```python
from build123d import *

# Parameters (mm, degrees)
BOSS_EXTRUDE1_DEPTH = 3.18
CUT_EXTRUDE1_DEPTH  = 3.18
SKETCH3_W           = 42
SKETCH3_H           = 20
CUT_EXTRUDE2_DEPTH  = 10
SKETCH4_R           = 2.2225
CUT_EXTRUDE3_DEPTH  = 10
SKETCH5_R           = 8.5
SKETCH5_W           = 12
SKETCH5_H           = 3.600941215
CUT_EXTRUDE4_DEPTH  = 10
SKETCH6_R           = 1.2
CUT_EXTRUDE5_DEPTH  = 10


with BuildPart() as part:
    # Sketch1 → Boss-Extrude1 (new body)
    with BuildSketch(Plane(origin=(0, 0, 0), x_dir=(1, 0, 0), z_dir=(0, 1, 0))):
        Polygon((12.7, 76.2), (-12.7, 76.2), (-12.7, 12.7), (-114.3, 12.7), (-114.3, -12.7), (-12.7, -12.7), (-12.7, -76.2), (12.7, -76.2), align=None)
    extrude(amount=BOSS_EXTRUDE1_DEPTH)

    # Sketch2 → Cut-Extrude1 (cut)
    with BuildSketch(Plane(origin=(0, 3.18, 0), x_dir=(1, 0, 0), z_dir=(0, 1, 0))):
        Polygon((-1.59, 73.02), (-1.59, 72.02), (-3.5, 72.02), (-3.5, 69.02), (-1.59, 69.02), (-1.59, 64.2), (1.59, 64.2), (1.59, 69.02), (3.5, 69.02), (3.5, 72.02), (1.59, 72.02), (1.59, 73.02), (5, 73.02), (5, 76.2), (-5, 76.2), (-5, 73.02), align=None)
        Polygon((1.59, -72.02), (3.5, -72.02), (3.5, -69.02), (1.59, -69.02), (1.59, -64.2), (-1.59, -64.2), (-1.59, -69.02), (-3.5, -69.02), (-3.5, -72.02), (-1.59, -72.02), (-1.59, -73.02), (-5, -73.02), (-5, -76.2), (5, -76.2), (5, -73.02), (1.59, -73.02), align=None)
    extrude(amount=-CUT_EXTRUDE1_DEPTH, mode=Mode.SUBTRACT)

    # Sketch3 → Cut-Extrude2 (cut)
    with BuildSketch(Plane(origin=(0, 0, 0), x_dir=(-1, 0, 0), z_dir=(0, -1, 0))):
        with Locations((78.3, 0)):
            Rectangle(SKETCH3_W, SKETCH3_H)
    extrude(amount=-CUT_EXTRUDE2_DEPTH, mode=Mode.SUBTRACT)

    # Sketch4 → Cut-Extrude3 (cut)
    with BuildSketch(Plane(origin=(0, 0, 0), x_dir=(-1, 0, 0), z_dir=(0, -1, 0))):
        with Locations((103.999, -5.2375)):
            Circle(SKETCH4_R)
        with Locations((103.999, 4.9225)):
            Circle(SKETCH4_R)
        with Locations((53.901, 4.9225)):
            Circle(SKETCH4_R)
        with Locations((53.901, -5.2375)):
            Circle(SKETCH4_R)
    extrude(amount=-CUT_EXTRUDE3_DEPTH, mode=Mode.SUBTRACT)

    # Sketch5 → Cut-Extrude4 (cut)
    with BuildSketch(Plane.XZ):
        with Locations((-37.467456586, 0.996077317)):
            Circle(SKETCH5_R)
        with Locations((-11.607456586, 0.996077317)):
            Circle(SKETCH5_R)
        with BuildLine():
            Line((-27.73362836, 10.446077317), (-21.33362836, 10.446077317))
            ThreePointArc((-21.33362836, 10.446077317), (-19.33362836, 8.446077317), (-21.33362836, 6.446077317))
            Line((-21.33362836, 6.446077317), (-27.73362836, 6.446077317))
            ThreePointArc((-27.73362836, 6.446077317), (-29.73362836, 8.446077317), (-27.73362836, 10.446077317))
        make_face()
        with Locations((-24.446347452, -7.921372698)):
            Rectangle(SKETCH5_W, SKETCH5_H)
    extrude(amount=-CUT_EXTRUDE4_DEPTH, mode=Mode.SUBTRACT)

    # Sketch6 → Cut-Extrude5 (cut)
    with BuildSketch(Plane(origin=(0, 3.18, 0), x_dir=(1, 0, 0), z_dir=(0, 1, 0))):
        with Locations((-3.437456586, -9.746077317)):
            Circle(SKETCH6_R)
        with Locations((-45.637456586, 7.753922683)):
            Circle(SKETCH6_R)
    extrude(amount=-CUT_EXTRUDE5_DEPTH, mode=Mode.SUBTRACT)


solid = part.part
```
Can you work these out from the model? Positions are in its coordinate system, mm. A direction names the side the tool comes from. Coordinates: 2 decimals unless noted, no trailing zeros. Order: outer loops, then holes, each group sorted by start corner. A loop starts at its lowest first (then second) coordinate and runs counter-clockwise, first axis right, second up.
1. If we section it at D-D (y = 2.7): Give the number of separate pieces and of enclosed holes in the cut face, then the cut area to 3 significant figures.
2. If we section it at B-B (z = -33): Please give me the cut outline in (x, y), then the cut area to 3 significant figures.
3. Thinking about a two-plate mould opening in X: for faces 1 (the face through (-12.7, 2, -45)), 2 (the face through (-9, 2, 76.2)), 3 (the face through (5, 2, -75)), 4 (the face through (-1.59, 2, 67)), which applies, +X half, -X half, draft (parallel to the pull), parting line (faces both ways), or undercut?
4. I need wall thicknesses on line 1 (X direction, y = 1, z = 1.5); line 2 (Z direction, x = -64.5, y = 2.7); line 3 (Z direction, x = 3, y = 0.3). Which ranges of each line are inside material? Lowest first, please.
5. For faces 5 (the face through (-3, 2, 73.02)), 6 (the face through (-5, 2, -75)), 7 (the face through (-78, 2, -10)), which set-ups out of +Z, -Z, +X, -X, +Y, -Y let a thin tool reach every point of the face, with its end or its side?
6. If we section it at C-C (x = -10): Please give me the cut outline in (y, z), then the cut area to 3 significant figures.
7. I'm going to push flat-ended pins straight in: pin 1 (1.5 mm diameter, centred on x = 2, y = 2, fed in from +Z); pin 2 (1 mm diameter, centred on x = -34.5, y = 1.5, fed in from +Z); pin 3 (1 mm diameter, centred on x = -0.5, y = 2, fed in from +Z). Where does each tip first touch, or does it pass through?
8. If we section it at A-A (x = -60): Please give me the cut outline in (y, z).
Entries:
1. separate pieces: 1
1. enclosed holes: 11
1. area: 4,860 mm2
2. outline: (-12.7, 0) - (12.7, 0) - (12.7, 3.18) - (-12.7, 3.18) - close
2. area: 80.8 mm2
3. face 1: -X half
3. face 2: draft
3. face 3: undercut
3. face 4: undercut
4. line 1: x = -114.3 to -99.3, -57.3 to -45.95, -28.98 to -20.09, -3.12 to 12.7
4. line 2: z = -12.7 to -10, 10 to 12.7
4. line 3: z = -73.02 to -72.02, -69.02 to 69.02, 72.02 to 73.02
5. face 5: +Z, +Y, -Y
5. face 6: -Z, +Y, -Y
5. face 7: +Y, -Y
6. outline: (0, -76.2) - (3.18, -76.2) - (3.18, -7.35) - (0, -7.35) - close; (0, 9.34) - (3.18, 9.34) - (3.18, 76.2) - (0, 76.2) - close
6. area: 432 mm2
7. pin 1: stops at z = 73.02
7. pin 2: stops at z = 12.7
7. pin 3: stops at z = 64.2
8. outline: (0, -12.7) - (3.18, -12.7) - (3.18, -10) - (0, -10) - close; (0, 10) - (3.18, 10) - (3.18, 12.7) - (0, 12.7) - close
